Here's how the part is built. I have some questions about the finished solid (model axes, mm). A direction names the side the tool comes from. Round coordinates to 2 decimals unless told otherwise and drop trailing zeros. Write each loop counter-clockwise with the first axis right and the second up, starting at its lowest first coordinate (ties: lowest second). Pieces come first, ordered by that corner, then holes. Notation, with made-up numbers: M 19.25,-24 L 43.25,-24 A21 cw 43.25,-8 Z; hole C 33.25,27.5 d7. An arc over 180 degrees is marked long. Use one line per item in the form item = value. Start each with the question number.
Q1. I want a section at A-A on z = -23. List the corners of the cut face in (x, y) for me, and give its area (3 significant figures).
Q2. I need wall thicknesses on line 1 along X through (y, z) = (3.25, -23); line 2 along X through (y, z) = (5.25, -17.5); line 3 along Y through (x, z) = (17, -5.75). Which ranges of each line are inside material? Lowest first, please. Write a range as from..to.
Q3. We'd pull the mould along Z, two halves only. Please class faces 4 (the face through (28.69, 5.07, -24.84)), 5 (the face through (13, 3, -33)), 6 (the face through (13.8, 2.6, -3.9)): +Z half, -Z half, draft (parallel to the pull), parting line (faces both ways), or undercut.
Q4. For faces 1 (the face through (33.4, 5.07, -0.57)), 2 (the face through (27.287, 4.93, -8.752)), 3 (the face through (5.502, 5.088, -3.944)), which set-ups out of +Z, -Z, +X, -X, +Y, -Y let a thin tool reach every point of the face, with its end or its side?
Q5. I want a section at B-B on y = 5. State how many separate pieces and enclosed holes the cut face has, and give its area (3 significant figures).
Q6. I want a section at D-D on z = -16. List the corners of the cut face in (x, y) for me, and give its area (3 significant figures).
Q7. I want a section at C-C on x = 4. List the corners of the cut face in (y, z) for me.
Q8. I'm going to push flat-ended pins straight in: pin 1 Ø8 at (x, z) = (27, -23) entering from +Y; pin 2 Ø1 at (x, y) = (6.5, 5) entering from +Z. Where does each tip first touch, or does it pass through?
```python
from build123d import *

# Parameters (mm, degrees)
SKETCH2_W           = 34
SKETCH2_H           = 33
BOSS_EXTRUDE1_DEPTH = 10
FILLET1_R           = 2
FILLET2_R           = 2
FILLET3_R           = 2
FILLET4_R           = 2
SKETCH3_R           = 2.5
CUT_EXTRUDE1_DEPTH  = 10
SKETCH4_W           = 28
SKETCH4_H           = 5
CUT_EXTRUDE2_DEPTH  = 10
FILLET5_R           = 2.5
FILLET6_R           = 2.5
SKETCH5_R           = 4
CUT_EXTRUDE3_DEPTH  = 60
SKETCH6_R           = 2
CUT_EXTRUDE4_DEPTH  = 10


with BuildPart() as part:
    # Sketch2 → Boss-Extrude1 (new body)
    with BuildSketch(Plane(origin=(0, 0, 0), x_dir=(1, 0, 0), z_dir=(0, 1, 0))):
        with Locations((17, 16.5)):
            Rectangle(SKETCH2_W, SKETCH2_H)
    extrude(amount=BOSS_EXTRUDE1_DEPTH)

    # Fillet1
    fillet1_edges = [part.edges().sort_by_distance(p)[0] for p in [
        (34, 5, 0),
    ]]
    fillet(fillet1_edges, radius=FILLET1_R)

    # Fillet2
    fillet2_edges = [part.edges().sort_by_distance(p)[0] for p in [
        (34, 5, -33),
    ]]
    fillet(fillet2_edges, radius=FILLET2_R)

    # Fillet3
    fillet3_edges = [part.edges().sort_by_distance(p)[0] for p in [
        (0, 5, -33),
    ]]
    fillet(fillet3_edges, radius=FILLET3_R)

    # Fillet4
    fillet4_edges = [part.edges().sort_by_distance(p)[0] for p in [
        (0, 5, 0),
    ]]
    fillet(fillet4_edges, radius=FILLET4_R)

    # Sketch3 → Cut-Extrude1 (cut)
    with BuildSketch(Plane(origin=(0, 10, 0), x_dir=(1, 0, 0), z_dir=(0, 1, 0))):
        with Locations(Location((7, 23, 0), (0, 0, 270))):
            Circle(SKETCH3_R)
        with Locations(Location((27, 23, 0), (0, 0, 270))):
            Circle(SKETCH3_R)
    extrude(amount=-CUT_EXTRUDE1_DEPTH, mode=Mode.SUBTRACT)

    # Sketch4 → Cut-Extrude2 (cut)
    with BuildSketch(Plane(origin=(0, 10, 0), x_dir=(1, 0, 0), z_dir=(0, 1, 0))):
        with Locations((14, 10.5)):
            Rectangle(SKETCH4_W, SKETCH4_H)
    extrude(amount=-CUT_EXTRUDE2_DEPTH, mode=Mode.SUBTRACT)

    # Fillet5
    fillet5_edges = [part.edges().sort_by_distance(p)[0] for p in [
        (28, 5, -13),
    ]]
    fillet(fillet5_edges, radius=FILLET5_R)

    # Fillet6
    fillet6_edges = [part.edges().sort_by_distance(p)[0] for p in [
        (28, 5, -8),
    ]]
    fillet(fillet6_edges, radius=FILLET6_R - 0.0001)  # a hair under: the kernel refuses the full size

    # Sketch5 → Cut-Extrude3 (cut)
    with BuildSketch(Plane.XY):
        with Locations((17, 5)):
            Circle(SKETCH5_R)
    extrude(amount=-CUT_EXTRUDE3_DEPTH, mode=Mode.SUBTRACT)

    # Sketch6 → Cut-Extrude4 (cut)
    with BuildSketch(Plane.XY):
        with Locations((7.5, 5)):
            Circle(SKETCH6_R)
    extrude(amount=-CUT_EXTRUDE4_DEPTH, mode=Mode.SUBTRACT)


solid = part.part
```
Reported:
q1.outline = M 0,0 L 4.5,0 L 4.5,10 L 0,10 Z; M 9.5,0 L 24.5,0 L 24.5,10 L 9.5,10 Z; M 29.5,0 L 34,0 L 34,10 L 29.5,10 Z; hole C 17,5 d8
q1.area = 190 mm^2
q2.line_1 = 0..4.5, 9.5..13.4, 20.6..24.5, 29.5..34
q2.line_2 = 0..13.01, 20.99..34
q2.line_3 = 0..1, 9..10
q3.face_4 = undercut
q3.face_5 = -Z half
q3.face_6 = draft
q4.face_1 = +Z, +X, +Y, -Y
q4.face_2 = -X, +Y, -Y
q4.face_3 = +Z
q5.separate_pieces = 4
q5.enclosed_holes = 2
q5.area = 686 mm^2
q6.outline = M 0,0 L 34,0 L 34,10 L 0,10 Z; hole C 17,5 d8
q6.area = 290 mm^2
q7.outline = M 0,-33 L 10,-33 L 10,-13 L 0,-13 Z; M 0,-8 L 10,-8 L 10,0 L 0,0 Z
q8.pin_1 = 10
q8.pin_2 = -13
